Verification items for this drawing (mm, ordinates from the low corner). A direction names the side the tool comes from. Coordinates: 2 decimals unless noted, no trailing zeros. Write each loop counter-clockwise with the first axis right and the second up, starting at its lowest first coordinate (ties: lowest second). Pieces come first, ordered by that corner, then holes. Notation, with made-up numbers: (-29, 0) -> (25, 0) arc R18 cw to (25, 5) -> close; hole circle Ø5 at (89, -29.75). An arc over 180 degrees is marked (long way). Answer as CSV lines item,"result".
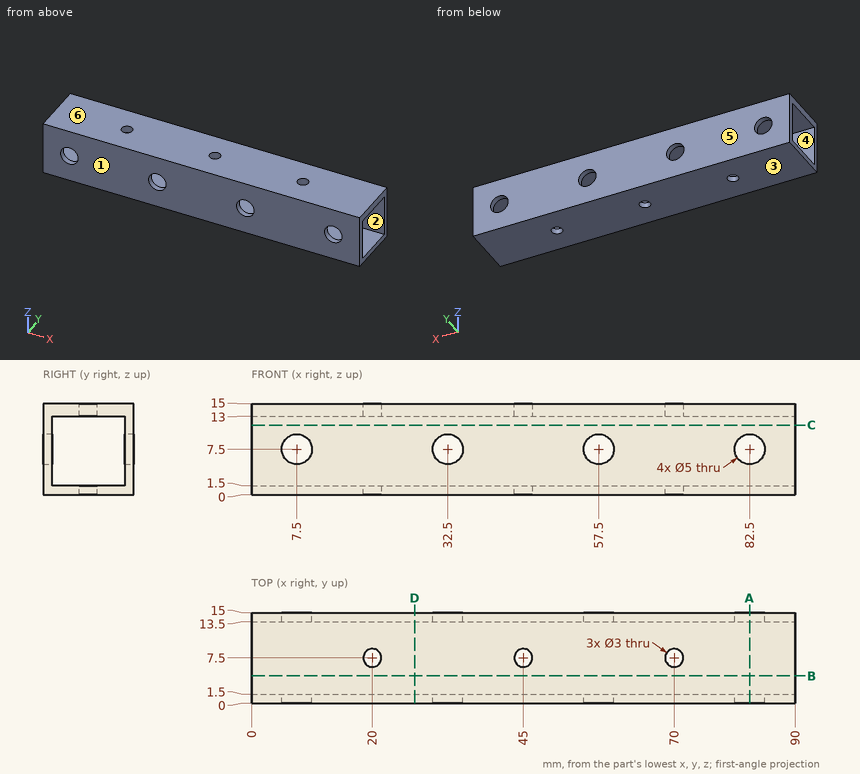
Item 1: Thickness scan on probe 1 along X at (y, z) = (14.1, 7.5); probe 2 along Y at (x, z) = (13, 7); probe 3 along Z at (x, y) = (66, 2). Record the ranges inside material, lowest first.
Responses:
probe 1,"x = 0 to 5, 10 to 30, 35 to 55, 60 to 80, 85 to 90"
probe 2,"y = 0 to 1.5, 13.5 to 15"
probe 3,"z = 0 to 1.5, 13 to 15"
Item 2: Cross-section at C-C, the plane z = 11.5. Record the cut outline in (x, y).
Responses:
outline,"(0, 0) -> (90, 0) -> (90, 1.5) -> (0, 1.5) -> close; (0, 13.5) -> (90, 13.5) -> (90, 15) -> (0, 15) -> close"
Item 3: Cross-section at A-A, the plane x = 82.5. Record the cut outline in (y, z), plus the area to 3 significant figures.
Responses:
outline,"(0, 0) -> (15, 0) -> (15, 5) -> (13.5, 5) -> (13.5, 1.5) -> (1.5, 1.5) -> (1.5, 5) -> (0, 5) -> close; (0, 10) -> (1.5, 10) -> (1.5, 13) -> (13.5, 13) -> (13.5, 10) -> (15, 10) -> (15, 15) -> (0, 15) -> close"
area,"72.0 mm2"
Item 4: Set-up check for the marked faces 1 and 2: record each of +Z, -Z, +X, -X, +Y, -Y from which the full face is reachable in a straight line by a thin tool's end or side.
Responses:
face 1,"+Z, -Z, +X, -X, -Y"
face 2,"+X, -X"
Item 5: Cross-section at D-D, the plane x = 27. Record the cut outline in (y, z).
Responses:
outline,"(0, 0) -> (15, 0) -> (15, 15) -> (0, 15) -> close; hole (1.5, 1.5) -> (13.5, 1.5) -> (13.5, 13) -> (1.5, 13) -> close"
Item 6: Release check for a two-part mould opening along Z. For the marked faces 3, 4, 5 and 6 record: +Z half, -Z half, draft (parallel to the pull), parting line (faces both ways), or undercut.
Responses:
face 3,"-Z half"
face 4,"undercut"
face 5,"draft"
face 6,"+Z half"
Item 7: Cross-section at B-B, the plane y = 4.5. Record the cut outline in (x, z).
Responses:
outline,"(0, 0) -> (90, 0) -> (90, 1.5) -> (0, 1.5) -> close; (0, 13) -> (90, 13) -> (90, 15) -> (0, 15) -> close"
